from build123d import *

# Parameters (mm, degrees)
EXTRUDE_1_DEPTH     = 455
SKETCH_3_R          = 2.1
CUT_EXTRUDE_1_DEPTH = 466.453246739
SKETCH_4_W          = 100
SKETCH_4_H          = 40
CUT_EXTRUDE_2_DEPTH = 466.453246739
SKETCH_5_R          = 2.605282574
CUT_EXTRUDE_3_DEPTH = 466.453246739


with BuildPart() as part:
    # 草图2 → 凸台-拉伸1 (new body)
    with BuildSketch(Plane.XY):
        Polygon((-98, -1), (-96.845299462, 1), (96.915299462, 1), (98.07, -1), align=None)
    extrude(amount=-EXTRUDE_1_DEPTH)

    # 草图3 → 切除-拉伸1 (cut, through all)
    with BuildSketch(Plane(origin=(0, -1, 0), x_dir=(-1, 0, 0), z_dir=(0, -1, 0))):
        with Locations(Location((78, 35, 0), (0, 0, 90))):
            Circle(SKETCH_3_R)
        with Locations(Location((78, 55, 0), (0, 0, 90))):
            Circle(SKETCH_3_R)
        with Locations(Location((-78, 55, 0), (0, 0, 270))):
            Circle(SKETCH_3_R)
        with Locations(Location((-78, 35, 0), (0, 0, 270))):
            Circle(SKETCH_3_R)
        with Locations(Location((-78, 420, 0), (0, 0, 90))):
            Circle(SKETCH_3_R)
        with Locations(Location((-78, 400, 0), (0, 0, 90))):
            Circle(SKETCH_3_R)
        with Locations(Location((78, 400, 0), (0, 0, 270))):
            Circle(SKETCH_3_R)
        with Locations(Location((78, 420, 0), (0, 0, 270))):
            Circle(SKETCH_3_R)
    extrude(amount=-CUT_EXTRUDE_1_DEPTH, mode=Mode.SUBTRACT)

    # 草图4 → 切除-拉伸2 (cut, through all)
    with BuildSketch(Plane.XZ.offset(1)):
        with Locations((0.035, -20)):
            Rectangle(SKETCH_4_W, SKETCH_4_H)
    extrude(amount=-CUT_EXTRUDE_2_DEPTH, mode=Mode.SUBTRACT)

    # 草图5 → 切除-拉伸3 (cut, through all)
    with BuildSketch(Plane.XZ.offset(1)):
        with Locations(Location((31.560145964, -260.175968549, 0), (0, 0, 270))):
            Circle(SKETCH_5_R)
        with Locations(Location((31.560145964, -268.040513613, 0), (0, 0, 270))):
            Circle(SKETCH_5_R)
        with Locations(Location((31.560145964, -275.759418954, 0), (0, 0, 270))):
            Circle(SKETCH_5_R)
        with Locations(Location((38.591431537, -263.539657654, 0), (0, 0, 270))):
            Circle(SKETCH_5_R)
        with Locations(Location((38.591431537, -273.011612977, 0), (0, 0, 270))):
            Circle(SKETCH_5_R)
        with Locations(Location((47.527390385, -268.469499033, 0), (0, 0, 270))):
            Circle(SKETCH_5_R)
        with Locations(Location((54.534326635, -263.539657654, 0), (0, 0, 270))):
            Circle(SKETCH_5_R)
        with Locations(Location((54.534326635, -273.011612977, 0), (0, 0, 270))):
            Circle(SKETCH_5_R)
        with Locations(Location((47.688259917, -277.526130321, 0), (0, 0, 270))):
            Circle(SKETCH_5_R)
        with Locations(Location((47.688259917, -259.038134333, 0), (0, 0, 270))):
            Circle(SKETCH_5_R)
        with Locations(Location((60.308400403, -258.8772648, 0), (0, 0, 270))):
            Circle(SKETCH_5_R)
        with Locations(Location((59.986661338, -277.526130321, 0), (0, 0, 270))):
            Circle(SKETCH_5_R)
    extrude(amount=-CUT_EXTRUDE_3_DEPTH, mode=Mode.SUBTRACT)


solid = part.part
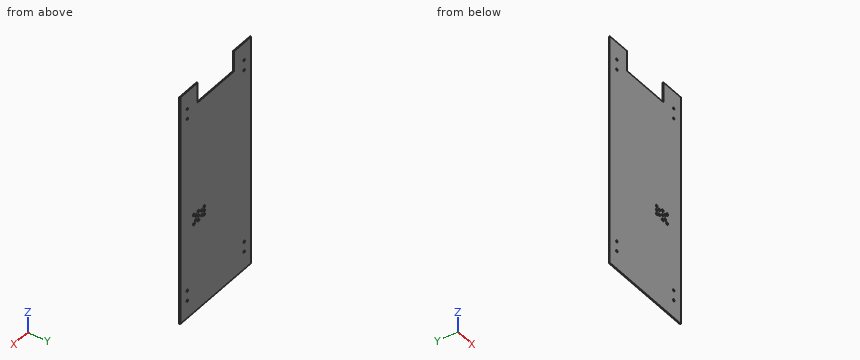
Source: CAD feature listing. Evaluate the final solid. Frame: model axes, mm. Give positions to 0.01 mm unless a question says otherwise; leave off trailing zeros. Loops run counter-clockwise (first coordinate to the right, second up) from the corner with the lowest first, then second, coordinate; pieces in that order, holes last. Notation, with made-up numbers: (-6.5, -14.75) -> (33.5, -14.75) arc R24 ccw to (33.5, 1.25) -> close; hole circle Ø9 at (48.5, 60.5). An arc over 180 degrees is marked (long way). Use a Markdown table: item, result. Add a question column.
1) Line query: line 1 along X through (y, z) = (-0.4, -55); line 2 along X through (y, z) = (0.1, -35) (3 decimals); line 3 along X through (y, z) = (0, -55). Output: solid intervals per line, ascending. Write a range as [from, to].
2) First-contact query: pin 1 (4.5 mm diameter, centred on x = 54.53, z = -263.54, fed in from -Y); pin 2 (1 mm diameter, centred on y = 0, z = -23.5, fed in from -X). Flat tips, straight axial feed; report the tip coordinate or a pass-through.
3) Section query B-B, the plane x = -28. Return the cut outline in (y, z), then the cut area to 3 significant figures.
4) Section query A-A, the plane y = -0.45. Count the separate pieces of the cut face and the enclosed holes in it, then the cut area to 3 significant figures.
Numbers:
| question | item | result |
|---|---|---|
| 1 | line 1 | x = [-97.65, -80.1], [-75.9, 75.9], [80.1, 97.72] |
| 1 | line 2 | x = [-97.365, -80.1], [-75.9, -49.965], [50.035, 75.9], [80.1, 97.435] |
| 1 | line 3 | x = [-97.42, -80.1], [-75.9, 75.9], [80.1, 97.49] |
| 2 | pin 1 | passes through |
| 2 | pin 2 | stops at x = -97.71 |
| 3 | outline | (-1, -455) -> (1, -455) -> (1, -40) -> (-1, -40) -> close |
| 3 | area | 830 mm2 |
| 4 | separate pieces | 1 |
| 4 | enclosed holes | 20 |
| 4 | area | 84,600 mm2 |
